Input: part model. Units: mm. Frame: model coordinates. Face numbers are marked on the shaded views. Round coordinates to 2 decimals unless told otherwise and drop trailing zeros. Loops run counter-clockwise (first coordinate to the right, second up) from the corner with the lowest first, then second, coordinate; pieces in that order, holes last.
(1) Cut plane B-B, the plane z = 2.5. Output: boundary loops of the cut face in (x, y).
(2) Cut plane A-A, the plane y = 0. Output: boundary loops of the cut face in (x, z), and give its area (3 significant figures).
(3) Draft query along X for the marked faces 1, 2 and 3. Return one class per face: released by +X, released by -X, zero draft, split by the parting line, or undercut.
(4) Cut plane D-D, the plane y = 1.5. Output: boundary loops of the cut face in (x, z).
(5) Line query: line 1 (Y direction, x = 0, z = 4.75); line 2 (Z direction, x = -10.25, y = 0.25); line 3 (X direction, y = -1.75, z = 5.25). Output: solid intervals per line, ascending.
(6) Cut plane C-C, the plane x = -5.5. Output: boundary loops of the cut face in (y, z), and give its area (3 significant figures).
(7) First-contact query: pin 1 Ø2.5 at (x, y) = (-10, 1) entering from +Z; pin 2 Ø4 at (x, y) = (4.5, 2) entering from +Z; pin 3 Ø2 at (x, z) = (10.5, 7) entering from +Y. Flat tips, straight axial feed; report the tip coordinate or a pass-through.
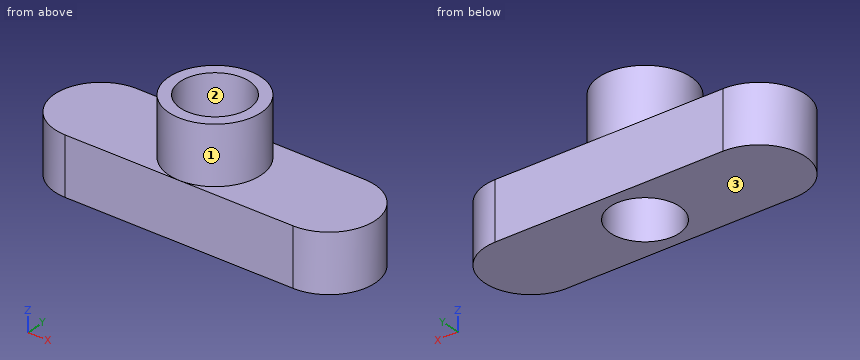
from build123d import *

# Parameters (mm, degrees)
SKETCH1_R           = 3
BOSS_EXTRUDE1_DEPTH = 5
SKETCH2_R           = 4
SKETCH2_R_2         = 3
BOSS_EXTRUDE2_DEPTH = 5


with BuildPart() as part:
    # Sketch1 → Boss-Extrude1 (new body)
    with BuildSketch(Plane.XY):
        with BuildLine():
            Line((-10, 4), (10, 4))
            ThreePointArc((10, 4), (14, 0), (10, -4))
            Line((10, -4), (-10, -4))
            ThreePointArc((-10, -4), (-14, 0), (-10, 4))
        make_face()
        Circle(SKETCH1_R, mode=Mode.SUBTRACT)
    extrude(amount=BOSS_EXTRUDE1_DEPTH)

    # Sketch2 → Boss-Extrude2 (add)
    with BuildSketch(Plane.XY.offset(5)):
        Circle(SKETCH2_R)
        Circle(SKETCH2_R_2, mode=Mode.SUBTRACT)
    extrude(amount=BOSS_EXTRUDE2_DEPTH)


solid = part.part
Reported:
1. outline: (-10, -4) - (10, -4) arc R4 ccw to (10, 4) - (-10, 4) arc R4 ccw to start; hole circle Ø6 at (0, 0)
2. outline: (-14, 0) - (-3, 0) - (-3, 10) - (-4, 10) - (-4, 5) - (-14, 5) - close; (3, 0) - (14, 0) - (14, 5) - (4, 5) - (4, 10) - (3, 10) - close
2. area: 120 mm2
3. face 1: split by the parting line
3. face 2: undercut
3. face 3: zero draft
4. outline: (-13.71, 0) - (-2.6, 0) - (-2.6, 10) - (-3.71, 10) - (-3.71, 5) - (-13.71, 5) - close; (2.6, 0) - (13.71, 0) - (13.71, 5) - (3.71, 5) - (3.71, 10) - (2.6, 10) - close
5. line 1: y = -4 to -3, 3 to 4
5. line 2: z = 0 to 5
5. line 3: x = -3.6 to -2.44, 2.44 to 3.6
6. outline: (-4, 0) - (4, 0) - (4, 5) - (-4, 5) - close
6. area: 40.0 mm2
7. pin 1: stops at z = 5
7. pin 2: stops at z = 10
7. pin 3: passes through
